Input: dimensioned drawing with shaded views. Units: mm. Origin: part minimum x, y, z. Coordinates: 2 decimals unless noted, no trailing zeros. Write each loop counter-clockwise with the first axis right and the second up, starting at its lowest first coordinate (ties: lowest second). Pieces come first, ordered by that corner, then holes. Notation, with made-up numbers: (0, 27.5) - (45, 27.5) arc R24 cw to (45, 60.5) - close; hole circle Ø7 at (-34.5, 36). An arc over 180 degrees is marked (long way). One line per question, with ' | ' between items.
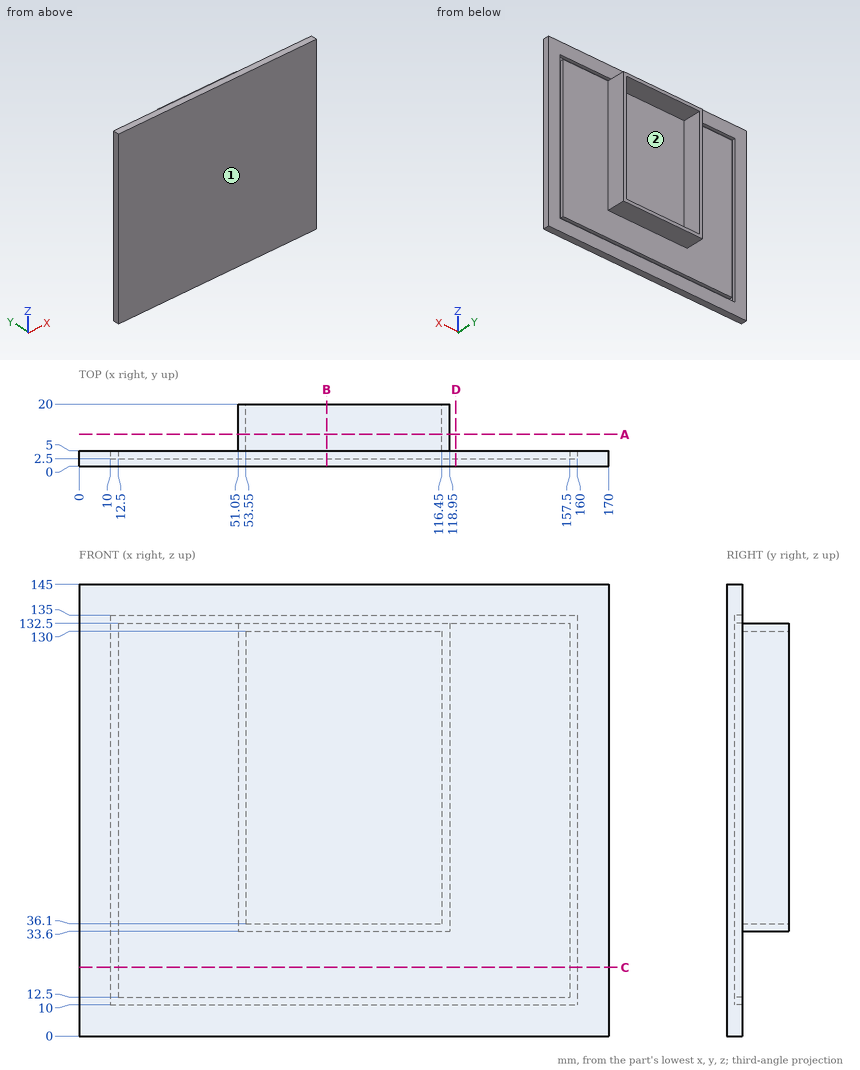
Item 1: Ray query, line 1 along X through (y, z) = (4.75, 125.5); line 2 along Z through (x, y) = (116, 7.75); line 3 along X through (y, z) = (11.75, 93). Return the intervals inside material, ascending. Write a range as [from, to].
Check sheet entries:
line 1: [0, 10], [12.5, 157.5], [160, 170] | line 2: [33.6, 36.1], [130, 132.5] | line 3: [51.05, 53.55], [116.45, 118.95]
Item 2: Cut plane B-B on x = 79.5. Return loops of the section in (y, z).
Check sheet entries:
outline: (0, 0) - (5, 0) - (5, 10) - (2.5, 10) - (2.5, 12.5) - (5, 12.5) - (5, 33.6) - (20, 33.6) - (20, 36.1) - (5, 36.1) - (5, 130) - (20, 130) - (20, 132.5) - (2.5, 132.5) - (2.5, 135) - (5, 135) - (5, 145) - (0, 145) - close
Item 3: Cut plane D-D on x = 121. Return loops of the section in (y, z), and give its area (4 significant figures).
Check sheet entries:
outline: (0, 0) - (5, 0) - (5, 10) - (2.5, 10) - (2.5, 12.5) - (5, 12.5) - (5, 132.5) - (2.5, 132.5) - (2.5, 135) - (5, 135) - (5, 145) - (0, 145) - close | area: 712.5 mm²
Item 4: Mould query, pull axis X, two halves, no side actions, for the marked faces 1 and 2. Classes: pulls with the +X half, pulls with the -X half, needs draft (parallel to the pull), parting line crosses it, or undercut.
Check sheet entries:
face 1: needs draft | face 2: undercut
Item 5: Cut plane A-A on y = 10.25. Return loops of the section in (x, z).
Check sheet entries:
outline: (51.05, 33.6) - (118.95, 33.6) - (118.95, 132.5) - (51.05, 132.5) - close; hole (53.55, 36.1) - (116.45, 36.1) - (116.45, 130) - (53.55, 130) - close
Item 6: Cut plane C-C on z = 22. Return loops of the section in (x, y).
Check sheet entries:
outline: (0, 0) - (170, 0) - (170, 5) - (160, 5) - (160, 2.5) - (157.5, 2.5) - (157.5, 5) - (12.5, 5) - (12.5, 2.5) - (10, 2.5) - (10, 5) - (0, 5) - close
Item 7: Pin query (flat end, axial travel): pin 1 Ø2 at (y, z) = (8, 83.5) entering from +X; pin 2 Ø1 at (x, z) = (21.5, 83) entering from +Y; pin 3 Ø12 at (y, z) = (14, 32.5) entering from -X; pin 4 Ø12 at (x, y) = (127, 14.5) entering from -Z. Return the tip coordinate at first contact, or that it passes through.
Check sheet entries:
pin 1: x = 118.95 | pin 2: y = 5 | pin 3: x = 51.05 | pin 4: through
